from build123d import *

# Parameters (mm, degrees)
SKETCH2_R           = 8.049775325
BOSS_EXTRUDE1_DEPTH = 19.05
SKETCH3_W           = 16.09955065
SKETCH3_H           = 32.199101299
BOSS_EXTRUDE2_DEPTH = 2.671544542
SKETCH4_W           = 63.40856
SKETCH4_H           = 19.05
BOSS_EXTRUDE3_DEPTH = 14.654134452
SKETCH5_W           = 19.05
SKETCH5_H           = 54.17415065
BOSS_EXTRUDE4_DEPTH = 1.128888889
SKETCH6_W           = 26.508568889
SKETCH6_H           = 19.05
BOSS_EXTRUDE5_DEPTH = 9.271057991


with BuildPart() as part:
    # Sketch2 → Boss-Extrude1 (new body)
    with BuildSketch(Plane.XY):
        with Locations(Location((0, 0, 0), (0, 0, 180))):
            Circle(SKETCH2_R)
    extrude(amount=BOSS_EXTRUDE1_DEPTH)

    # Sketch3 → Boss-Extrude2 (add)
    with BuildSketch(Plane(origin=(0, 0, 0), x_dir=(-1, 0, 0), z_dir=(0, 0, -1))):
        with Locations((0, 16.099550649)):
            Rectangle(SKETCH3_W, SKETCH3_H)
    extrude(amount=-BOSS_EXTRUDE2_DEPTH)

    # Sketch4 → Boss-Extrude3 (add)
    with BuildSketch(Plane(origin=(0, 32.199101299, 0), x_dir=(1, 0, 0), z_dir=(0, 1, 0))):
        with Locations((0, -9.525)):
            Rectangle(SKETCH4_W, SKETCH4_H)
    extrude(amount=BOSS_EXTRUDE3_DEPTH)

    # Sketch5 → Boss-Extrude4 (add)
    with BuildSketch(Plane(origin=(31.70428, 0, 0), x_dir=(0, 0, -1), z_dir=(1, 0, 0))):
        with Locations((-9.525, 59.286176624)):
            Rectangle(SKETCH5_W, SKETCH5_H)
    boss_extrude4 = extrude(amount=BOSS_EXTRUDE4_DEPTH)

    # Mirror1: Boss-Extrude4 across plane
    add(boss_extrude4.mirror(Plane(origin=(0, 0, 0), x_dir=(0, 0, 1), z_dir=(1, 0, 0))))

    # Sketch6 → Boss-Extrude5 (add)
    with BuildSketch(Plane(origin=(0, 86.373251949, 0), x_dir=(1, 0, 0), z_dir=(0, 1, 0))):
        with Locations((19.578884444, -9.525)):
            Rectangle(SKETCH6_W, SKETCH6_H)
    boss_extrude5 = extrude(amount=BOSS_EXTRUDE5_DEPTH)

    # Mirror2: Boss-Extrude4, Boss-Extrude5 across plane
    add(boss_extrude4.mirror(Plane(origin=(0, 0, 0), x_dir=(0, 0, 1), z_dir=(1, 0, 0))))
    add(boss_extrude5.mirror(Plane(origin=(0, 0, 0), x_dir=(0, 0, 1), z_dir=(1, 0, 0))))


solid = part.part
The model under review builds one solid part; all positions refer to its coordinate system, in mm. A direction names the side the tool comes from. Coordinates: 2 decimals unless noted, no trailing zeros. Loops run counter-clockwise (first coordinate to the right, second up) from the corner with the lowest first, then second, coordinate; pieces in that order, holes last.
(1) Insertion check: P1, Ø2, axis at y = 6, z = 3, coming from the -X side; P2, Ø9.5, axis at x = -13, z = 6, coming from the -Y side; P3, Ø5, axis at x = -5, z = 4.5, coming from the -Y side. Each pin has a flat end and moves straight along its axis. Give the tip position at first contact, or say it passes through.
Determined:
P1: stops at x = -8.05
P2: stops at y = 32.2
P3: stops at y = -7.65
(2) Wall thickness on L1, parallel to Y at x = 8.5, z = 12.75; L2, parallel to X at y = 76, z = 8.75; L3, parallel to Y at x = 5.5, z = 11.5: over which ranges is each line inside the solid? List them lowest first.
Determined:
L1: y = 32.2 to 46.85, 86.37 to 95.64
L2: x = -32.83 to -31.7, 31.7 to 32.83
L3: y = -5.88 to 5.88, 32.2 to 46.85
(3) Consider section C-C, the plane y = 50.5. Give the boundary of the cut face in (x, z), plus the area to 3 significant figures.
Determined:
outline: (-32.83, 0) - (-31.7, 0) - (-31.7, 19.05) - (-32.83, 19.05) - close; (31.7, 0) - (32.83, 0) - (32.83, 19.05) - (31.7, 19.05) - close
area: 43.0 mm2
(4) Consider section D-D, the plane x = 0. Give the boundary of the cut face in (y, z), plus the area to 3 significant figures.
Determined:
outline: (-8.05, 0) - (46.85, 0) - (46.85, 19.05) - (32.2, 19.05) - (32.2, 2.67) - (8.05, 2.67) - (8.05, 19.05) - (-8.05, 19.05) - close
area: 650 mm2
(5) Draft analysis for pull direction X (two halves, no side actions). For faces 5 (the flat face through (-32.833, 63, 10)), 6 (the cylindrical face through (1.05, -7.98, 9.39)), 7 (the flat face through (-19, 86.373, 9)), state which applies: +X half, -X half, draft (parallel to the pull), parting line (faces both ways), or undercut.
Determined:
face 5: -X half
face 6: parting line
face 7: undercut
(6) Consider section A-A, the plane x = -21. Give the boundary of the cut face in (y, z).
Determined:
outline: (32.2, 0) - (46.85, 0) - (46.85, 19.05) - (32.2, 19.05) - close; (86.37, 0) - (95.64, 0) - (95.64, 19.05) - (86.37, 19.05) - close
(7) Consider section B-B, the plane z = 4.75. Give the boundary of the cut face in (x, y).
Determined:
outline: (-32.83, 32.2) - (32.83, 32.2) - (32.83, 95.64) - (6.32, 95.64) - (6.32, 86.37) - (31.7, 86.37) - (31.7, 46.85) - (-31.7, 46.85) - (-31.7, 86.37) - (-6.32, 86.37) - (-6.32, 95.64) - (-32.83, 95.64) - close; circle Ø16.1 at (0, 0)
(8) Tool access review of faces 1 (the flat face through (31.704, 67, 10)), 2 (the flat face through (-8.05, 16, 1)), 3 (the flat face through (8.05, 16, 1)), 4 (the flat face through (-6.325, 91, 10)): name each direction out of +Z, -Z, +X, -X, +Y, -Y from which nothing blocks a thin tool from reaching the whole face with its end or side.
Determined:
face 1: +Z, -Z
face 2: +Z, -Z, -X, -Y
face 3: +Z, -Z, +X, -Y
face 4: +Z, -Z, +Y
